Here's how the part is built. I have some questions about the finished solid (model axes, mm). Face numbers are marked on the shaded views. A direction names the side the tool comes from. Coordinates: 2 decimals unless noted, no trailing zeros. Answer as a JSON object with one key per item and string values. Group by question number.
1) I need wall thicknesses on probe 1 along X at (y, z) = (30.5, 11.5); probe 2 along X at (y, z) = (6, 5); probe 3 along Y at (x, z) = (37.5, 30.5) (3 decimals). Which ranges of each line are inside material? Lowest first, please. Write a range as [from, to].
2) I'm going to push flat-ended pins straight in: pin 1 (5.5 mm diameter, centred on x = 85.19, y = 15, fed in from -Z); pin 2 (2 mm diameter, centred on y = 22, z = 31, fed in from +X); pin 3 (3.5 mm diameter, centred on x = 0, y = -3.5, fed in from +Z); pin 4 (2 mm diameter, centred on x = 21, y = 60, fed in from +Z). Where does each tip first touch, or does it pass through?
3) Which directions (+Z, -Z, +X, -X, +Y, -Y) give clear straight access to the entire face, cutting with the end or side of a thin tool? Please do the marked faces 4, 5 and 6.
4) If we mould it in two halves opening along X, with no side actions, what happens to the marked faces 1, 2 and 3? For each: +X half, -X half, draft (parallel to the pull), parting line (faces both ways), or undercut.
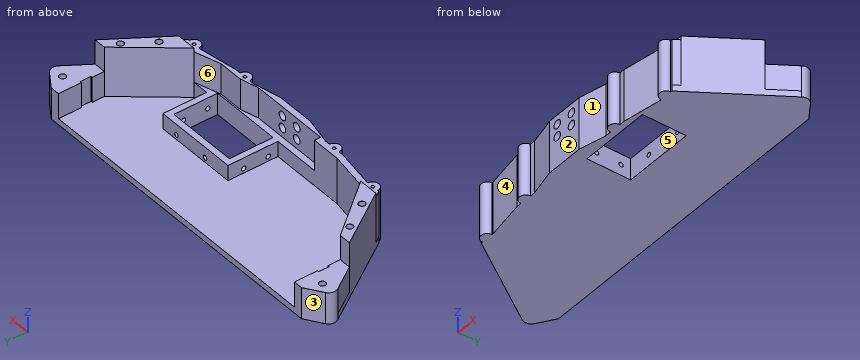
```python
from build123d import *

# Parameters (mm, degrees)
EXTRUDE_1_DEPTH                  = 4
EXTRUDE_2_DEPTH                  = 16.5
SKETCH_4_W                       = 46.6
SKETCH_4_H                       = 28.6
CUT_EXTRUDE_1_DEPTH              = 4
EXTRUDE_3_DEPTH                  = 10
HOLE_WIZARD_M2_5_1_D             = 2.9
HOLE_WIZARD_M2_5_1_CSINK_D       = 2.95
HOLE_WIZARD_M2_5_1_CSINK_ANGLE   = 90
HOLE_WIZARD_M2_5_2_D             = 2.9
HOLE_WIZARD_M2_5_2_CSINK_D       = 2.95
HOLE_WIZARD_M2_5_2_CSINK_ANGLE   = 90
HOLE_WIZARD_M5_1_D               = 4.2
HOLE_WIZARD_M5_1_DEPTH           = 5
HOLE_WIZARD_M5_1_CSINK_D         = 4.25
HOLE_WIZARD_M5_1_CSINK_ANGLE     = 90
HOLE_WIZARD_M5_1_TIP             = 1.2618073
EXTRUDE_4_DEPTH                  = 17
EXTRUDE_START                    = -17
EXTRUDE_5_DEPTH                  = 34
EXTRUDE_6_DEPTH                  = 20
SKETCH_20_W                      = 52
SKETCH_20_H                      = 4
CUT_EXTRUDE_2_DEPTH              = 3
CUT_EXTRUDE_3_DEPTH              = 10
SKETCH_22_R                      = 4
EXTRUDE_7_DEPTH                  = 34
HOLE_WIZARD_M2_5_1_2_D           = 2.05
HOLE_WIZARD_M2_5_1_2_DEPTH       = 10
HOLE_WIZARD_M2_5_1_2_CSINK_D     = 2.1
HOLE_WIZARD_M2_5_1_2_CSINK_ANGLE = 90
HOLE_WIZARD_M2_5_1_2_TIP         = 0.615882135
CUT_EXTRUDE_4_DEPTH              = 20
EXTRUDE_8_DEPTH                  = 32.5
HOLE_WIZARD_M5_2_D               = 4.2
HOLE_WIZARD_M5_2_DEPTH           = 10
HOLE_WIZARD_M5_2_CSINK_D         = 4.25
HOLE_WIZARD_M5_2_CSINK_ANGLE     = 90
HOLE_WIZARD_M5_2_TIP             = 1.2618073
FILLET_1_R                       = 5
HOLE_WIZARD_M5_1_2_D             = 5.5
HOLE_WIZARD_M5_1_2_DEPTH         = 10
HOLE_WIZARD_M5_1_2_CSINK_D       = 5.55
HOLE_WIZARD_M5_1_2_CSINK_ANGLE   = 90
HOLE_WIZARD_M5_1_2_TIP           = 1.652366702


with BuildPart() as part:
    # 草图2 → 凸台-拉伸1 (new body)
    with BuildSketch(Plane.XY):
        Polygon((80, 0), (-80, 0), (-120, 60), (-105, 70), (105, 70), (120, 60), align=None)
    extrude(amount=EXTRUDE_1_DEPTH)

    # 草图3 → 凸台-拉伸2 (add)
    with BuildSketch(Plane.XY.offset(4)):
        Polygon((105, 70), (99, 70), (99, 55), (100, 55), (100, 48), (99, 48), (99, 40), (106.666666667, 40), (120, 60), align=None)
        Polygon((-120, 60), (-105, 70), (-99, 70), (-99, 55), (-100, 55), (-100, 48), (-99, 48), (-99, 40), (-106.666666667, 40), align=None)
    extrude(amount=EXTRUDE_2_DEPTH)

    # 草图4 → 切除-拉伸1 (cut)
    with BuildSketch(Plane.XY.offset(4)):
        with Locations((32, 14.3)):
            Rectangle(SKETCH_4_W, SKETCH_4_H)
    extrude(amount=-CUT_EXTRUDE_1_DEPTH, mode=Mode.SUBTRACT)

    # 草图5 → 凸台-拉伸3 (add)
    with BuildSketch(Plane.XY.offset(4)):
        Polygon((55.3, 28.6), (55.3, 0), (80, 0), (82.666666667, 4), (59.3, 4), (59.3, 32.6), (4.7, 32.6), (4.7, 4), (-82.666666667, 4), (-80, 0), (8.7, 0), (8.7, 28.6), align=None)
    extrude(amount=EXTRUDE_3_DEPTH)

    # Hole Wizard M2.5 _1 (through all)
    with Locations(Plane(origin=(0, 32.6, 0), x_dir=(1, 0, 0), z_dir=(0, 1, 0))):
        with Locations((24, -7), (48, -7)):
            CounterSinkHole(HOLE_WIZARD_M2_5_1_D / 2, HOLE_WIZARD_M2_5_1_CSINK_D / 2, counter_sink_angle=HOLE_WIZARD_M2_5_1_CSINK_ANGLE)

    # M2.5 间隙孔2 (through all)
    with Locations(Plane.ZY.offset(-4.7)):
        with Locations((7, 22.3), (7, 6.3)):
            CounterSinkHole(HOLE_WIZARD_M2_5_2_D / 2, HOLE_WIZARD_M2_5_2_CSINK_D / 2, counter_sink_angle=HOLE_WIZARD_M2_5_2_CSINK_ANGLE)

    # Hole Wizard M5 _1
    with Locations(Plane.XY.offset(20.5)):
        with Locations((-109, 59.5), (109, 59.5)):
            CounterSinkHole(HOLE_WIZARD_M5_1_D / 2, HOLE_WIZARD_M5_1_CSINK_D / 2, depth=HOLE_WIZARD_M5_1_DEPTH, counter_sink_angle=HOLE_WIZARD_M5_1_CSINK_ANGLE)
            with Locations((0, 0, -(HOLE_WIZARD_M5_1_DEPTH + HOLE_WIZARD_M5_1_TIP / 2))):  # 118° drill point
                Cone(0, HOLE_WIZARD_M5_1_D / 2, HOLE_WIZARD_M5_1_TIP, mode=Mode.SUBTRACT)

    # 草图16 → 凸台-拉伸4 (add)
    with BuildSketch(Plane(origin=(0, 0, 0), x_dir=(-1, 0, 0), z_dir=(0, 0, -1))):
        Polygon((-70, 0), (-45, -4), (45, -4), (70, 0), align=None)
    extrude(amount=-EXTRUDE_4_DEPTH)

    # 草图17 → 凸台-拉伸5 (add)
    with BuildSketch(Plane.XY.offset(17).offset(EXTRUDE_START)):
        Polygon((-30, -4), (-12.5, -8), (12.5, -8), (30, -4), align=None)
    extrude(amount=EXTRUDE_5_DEPTH)

    # 草图19 → 凸台-拉伸6 (add)
    with BuildSketch(Plane.XY.offset(14)):
        Polygon((-78.666666667, 4), (-82.666666667, 4), (-80, 0), (-70, 0), (-45, -4), (-26, -4), (-26, 0), (-45, 0), (-70, 4), align=None)
        Polygon((45, 0), (26, 0), (26, -4), (45, -4), (70, 0), (80, 0), (82.666666667, 4), (78.666666667, 4), (70, 4), align=None)
    extrude(amount=EXTRUDE_6_DEPTH)

    # 草图20 → 切除-拉伸2 (cut)
    with BuildSketch(Plane.XY.offset(17)):
        with Locations((0, -2)):
            Rectangle(SKETCH_20_W, SKETCH_20_H)
    extrude(amount=-CUT_EXTRUDE_2_DEPTH, mode=Mode.SUBTRACT)

    # 草图21 → 切除-拉伸3 (cut)
    with BuildSketch(Plane.XY.offset(14)):
        Polygon((4.7, 4), (4.7, 0), (-45, 0), (-70, 4), align=None)
    extrude(amount=-CUT_EXTRUDE_3_DEPTH, mode=Mode.SUBTRACT)

    # 草图22 → 凸台-拉伸7 (add)
    with BuildSketch(Plane.XY.offset(34)):
        with Locations((-75, 0)):
            Circle(SKETCH_22_R)
        with Locations((-37.5, -4)):
            Circle(SKETCH_22_R)
        with Locations((37.5, -4)):
            Circle(SKETCH_22_R)
        with Locations((75, 0)):
            Circle(SKETCH_22_R)
    extrude(amount=-EXTRUDE_7_DEPTH)

    # Hole Wizard M2.5 _1 2
    with Locations(Plane.XY.offset(34)):
        with Locations((-75, 0), (-37.5, -4), (37.5, -4), (75, 0)):
            CounterSinkHole(HOLE_WIZARD_M2_5_1_2_D / 2, HOLE_WIZARD_M2_5_1_2_CSINK_D / 2, depth=HOLE_WIZARD_M2_5_1_2_DEPTH, counter_sink_angle=HOLE_WIZARD_M2_5_1_2_CSINK_ANGLE)
            with Locations((0, 0, -(HOLE_WIZARD_M2_5_1_2_DEPTH + HOLE_WIZARD_M2_5_1_2_TIP / 2))):  # 118° drill point
                Cone(0, HOLE_WIZARD_M2_5_1_2_D / 2, HOLE_WIZARD_M2_5_1_2_TIP, mode=Mode.SUBTRACT)

    # 草图25 → 切除-拉伸4 (cut)
    with BuildSketch(Plane.XY.offset(34)):
        Polygon((26, 0), (26, -4), (37.515153504, -1), (53.499458489, -1), (70, 4), (45, 0), align=None)
    extrude(amount=-CUT_EXTRUDE_4_DEPTH, mode=Mode.SUBTRACT)

    # 草图26 → 凸台-拉伸8 (add)
    with BuildSketch(Plane.XY.offset(4)):
        Polygon((-99, 40), (-106.666666667, 40), (-82.666666667, 4), (-70, 4), align=None)
        Polygon((82.666666667, 4), (70, 4), (99, 40), (106.666666667, 40), align=None)
    extrude(amount=EXTRUDE_8_DEPTH)

    # M5 螺纹孔的螺纹孔钻头2
    with Locations(Plane.XY.offset(36.5)):
        with Locations((-96.286602224, 31.641005887), (-85.192598299, 15), (85.192598299, 15), (96.286602224, 31.641005887)):
            CounterSinkHole(HOLE_WIZARD_M5_2_D / 2, HOLE_WIZARD_M5_2_CSINK_D / 2, depth=HOLE_WIZARD_M5_2_DEPTH, counter_sink_angle=HOLE_WIZARD_M5_2_CSINK_ANGLE)
            with Locations((0, 0, -(HOLE_WIZARD_M5_2_DEPTH + HOLE_WIZARD_M5_2_TIP / 2))):  # 118° drill point
                Cone(0, HOLE_WIZARD_M5_2_D / 2, HOLE_WIZARD_M5_2_TIP, mode=Mode.SUBTRACT)

    # 圆角1
    fillet_1_edges = [part.edges().sort_by_distance(p)[0] for p in [
        (120, 60, 10.25),
        (-120, 60, 10.25),
    ]]
    fillet(fillet_1_edges, radius=FILLET_1_R)

    # Hole Wizard M5 _1 2
    with Locations(Plane(origin=(0, -4, 0), x_dir=(1, 0, 0), z_dir=(0, 1, 0))):
        with Locations((-6, -20), (6, -20), (6, -28), (-6, -28)):
            CounterSinkHole(HOLE_WIZARD_M5_1_2_D / 2, HOLE_WIZARD_M5_1_2_CSINK_D / 2, depth=HOLE_WIZARD_M5_1_2_DEPTH, counter_sink_angle=HOLE_WIZARD_M5_1_2_CSINK_ANGLE)
            with Locations((0, 0, -(HOLE_WIZARD_M5_1_2_DEPTH + HOLE_WIZARD_M5_1_2_TIP / 2))):  # 118° drill point
                Cone(0, HOLE_WIZARD_M5_1_2_D / 2, HOLE_WIZARD_M5_1_2_TIP, mode=Mode.SUBTRACT)


solid = part.part
```
Determined:
{
 "1": {"probe 1": "[-100.33, -91.35], [4.7, 59.3], [91.35, 100.33]", "probe 2": "[-84, -71.61], [4.7, 8.7], [55.3, 59.3], [71.61, 84]", "probe 3": "[-8, -5.025], [-2.975, -1.004]"},
 "2": {"pin 1": "z = 0", "pin 2": "x = 95.33", "pin 3": "z = 34", "pin 4": "z = 4"},
 "3": {"face 4": "+Z, -Z, -Y", "face 5": "+Z, -Z", "face 6": "+Z, +Y"},
 "4": {"face 1": "undercut", "face 2": "draft", "face 3": "-X half"}
}
